```python
from build123d import *

# Parameters (mm, degrees)
EXTRUDE_2_DEPTH         = 20
SKETCH_3_R              = 1.65
CUT_EXTRUDE_2_DEPTH     = 20
DELETE_FACE_1_OUTLINE_R = 1.65
DELETE_FACE_1_DEPTH     = 20


# Read off the part's stored shape, not the designer's step: 删除面1
with BuildPart() as part:
    # 草图1 → 凸台-拉伸2 (new body)
    with BuildSketch(Plane.XY):
        with BuildLine():
            Line((-20, -21), (0, -21))
            ThreePointArc((0, -21), (-21, 0), (0, 21))
            Line((0, 21), (0, 29))
            ThreePointArc((0, 29), (-26.925824036, 10.770329614), (-20, -21))
        make_face()
    extrude(amount=EXTRUDE_2_DEPTH)

    # 草图3 → 切除-拉伸2 (cut)
    with BuildSketch(Plane.XY):
        with Locations((-12.5, 21.650635095)):
            Circle(SKETCH_3_R)
        with Locations((-21.650635095, 12.5)):
            Circle(SKETCH_3_R)
        with Locations((-21.650635095, -12.5)):
            Circle(SKETCH_3_R)
    extrude(amount=CUT_EXTRUDE_2_DEPTH, mode=Mode.SUBTRACT)

    # Delete Face 1 outline → Delete Face 1 (add)
    with BuildSketch(Plane.XY):
        with Locations((-12.5, 21.650635095)):
            Circle(DELETE_FACE_1_OUTLINE_R)
    extrude(amount=DELETE_FACE_1_DEPTH)


solid = part.part
```
Can you work these out from the model? Positions are in its coordinate system, mm. Coordinates: 2 decimals unless noted, no trailing zeros. Order: outer loops, then holes, each group sorted by start corner. A loop starts at its lowest first (then second) coordinate and runs counter-clockwise, first axis right, second up. Notation, with made-up numbers: (60.5, 12) - (84.5, 12) arc R30 ccw to (84.5, 38) - close; hole circle Ø9 at (50.25, -6). An arc over 180 degrees is marked (long way). Answer in a Markdown table with one row per item.
1. Suppose I cut it at C-C (y = 13). Please give me the cut outline in (x, z).
Reply:
| item | result |
|---|---|
| outline | (-25.92, 0) - (-23.22, 0) - (-23.22, 20) - (-25.92, 20) - close; (-20.08, 0) - (-16.49, 0) - (-16.49, 20) - (-20.08, 20) - close |
2. If I drill on line 1 along Y through (x, z) = (-7.5, 8.5); line 2 along Y through (x, z) = (-12, 15); line 3 along X through (y, z) = (13.5, 13.5), over which ranges is the centre line in solid material (lowest first)?
Reply:
| item | result |
|---|---|
| line 1 | y = -21 to -19.62, 19.62 to 28.01 |
| line 2 | y = -21 to -17.23, 17.23 to 26.4 |
| line 3 | x = -25.67 to -22.96, -20.34 to -16.09 |
3. For pin 1 (1 mm diameter, centred on y = -11.5, z = 8.5, fed in from +X); pin 2 (1 mm diameter, centred on y = 2.5, z = 9, fed in from +X); pin 3 (8 mm diameter, centred on y = 20, z = 2.5, fed in from -X), each with a flat end and sliding along its axis, tell me the tip position at first contact or that it passes through.
Reply:
| item | result |
|---|---|
| pin 1 | stops at x = -17.23 |
| pin 2 | stops at x = -20.78 |
| pin 3 | stops at x = -24.19 |
4. Suppose I cut it at B-B (x = -3.25). Please give me the cut outline in (y, z), and give its area (3 significant figures).
Reply:
| item | result |
|---|---|
| outline | (-21, 0) - (-20.75, 0) - (-20.75, 20) - (-21, 20) - close; (20.75, 0) - (28.82, 0) - (28.82, 20) - (20.75, 20) - close |
| area | 166 mm^2 |
5. Suppose I cut it at D-D (y = 0). Please give me the cut outline in (x, z).
Reply:
| item | result |
|---|---|
| outline | (-29, 0) - (-21, 0) - (-21, 20) - (-29, 20) - close |
6. Suppose I cut it at A-A (z = 6.75). Please give me the cut outline in (x, y).
Reply:
| item | result |
|---|---|
| outline | (-20, -21) - (0, -21) arc R21 cw to (0, 21) - (0, 29) arc R29 ccw to start; hole circle Ø3.3 at (-21.65, -12.5); hole circle Ø3.3 at (-21.65, 12.5) |
7. If we mould it in two halves opening along X, with no side actions, what happens to faces 1 (the flat face through (-21, 4, 0)), 2 (the cylindrical face through (-20.126, -13.132, 9.86)), 3 (the flat face through (0, 25, 10))? For each: pulls with the +X half, pulls with the -X half, needs draft (parallel to the pull), parting line crosses it, or undercut.
Reply:
| item | result |
|---|---|
| face 1 | needs draft |
| face 2 | undercut |
| face 3 | pulls with the +X half |
